Here's the drawing with two shaded views (mm, measured from the low corner). I have some questions. Round coordinates to 2 decimals unless told otherwise and drop trailing zeros. Loops run counter-clockwise (first coordinate to the right, second up) from the corner with the lowest first, then second, coordinate; pieces in that order, holes last. Notation, with made-up numbers: (54.25, 2) -> (105.25, 2) arc R26 cw to (105.25, 23) -> close; hole circle Ø3 at (10.25, 48.25). An arc over 180 degrees is marked (long way). Write item = value, one per line.
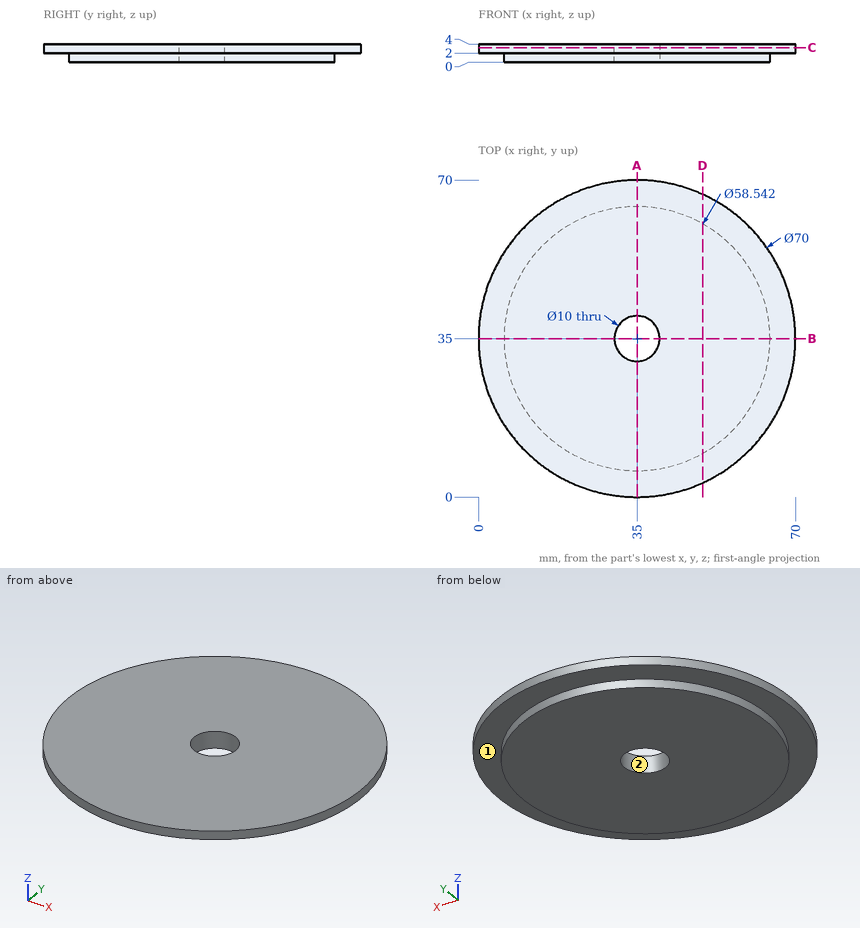
1. Suppose I cut it at A-A, the plane x = 35. List the corners of the cut face in (y, z) for me, and give its area (3 significant figures).
Entries:
outline = (0, 2) -> (5.73, 2) -> (5.73, 0) -> (30, 0) -> (30, 4) -> (0, 4) -> close; (40, 0) -> (64.27, 0) -> (64.27, 2) -> (70, 2) -> (70, 4) -> (40, 4) -> close
area = 217 mm²
2. I need wall thicknesses on line 1 (Y direction, x = 35, z = 1.3); line 2 (Y direction, x = 35, z = 2.1); line 3 (Z direction, x = 11, y = 16). Which ranges of each line are inside material? Lowest first, please. Write a range as [from, to].
Entries:
line_1 = [5.73, 30], [40, 64.27]
line_2 = [0, 30], [40, 70]
line_3 = [2, 4]
3. Suppose I cut it at C-C, the plane z = 3.2. List the corners of the cut face in (x, y) for me, and give its area (3 significant figures).
Entries:
outline = circle Ø70 at (35, 35); hole circle Ø10 at (35, 35)
area = 3,770 mm²
4. I'm going to push a flat-ended pin straight in: pin 1 (2 mm diameter, centred on y = 22, z = 2, fed in from -X). Where does the tip first touch, or does it pass through?
Entries:
pin_1 = 2.12
5. We'd pull the mould along X, two halves only. Please class the marked faces 1 and 2: released by +X, released by -X, zero draft, split by the parting line, or undercut.
Entries:
face_1 = zero draft
face_2 = undercut
6. Suppose I cut it at D-D, the plane x = 49.5. List the corners of the cut face in (y, z) for me (3 decimals).
Entries:
outline = (3.145, 2) -> (9.573, 2) -> (9.573, 0) -> (60.427, 0) -> (60.427, 2) -> (66.855, 2) -> (66.855, 4) -> (3.145, 4) -> close
